Read the model definition and answer for the solid it produces. Units are mm, in the model's axes. A direction names the side the tool comes from. Give positions to 0.01 mm unless a question says otherwise; leave off trailing zeros. Order: outer loops, then holes, each group sorted by start corner. A loop starts at its lowest first (then second) coordinate and runs counter-clockwise, first axis right, second up. Notation, with made-up numbers: M 17,86 L 30,86 A20 ccw 30,109 Z; hole C -35,-11 d11. An arc over 180 degrees is marked long. Write item = value, one per line. Start each with the question number.
from build123d import *

# Parameters (mm, degrees)
SKETCH1_R           = 38.1
SKETCH1_R_2         = 34.671
BOSS_EXTRUDE1_DEPTH = 12.7
SKETCH2_W           = 12.7
SKETCH2_H           = 12.7
BOSS_EXTRUDE2_DEPTH = 12.7
SKETCH4_W           = 2.54
SKETCH4_H           = 58.988343485
CUT_EXTRUDE2_DEPTH  = 65.340360647
BOSS_EXTRUDE3_REACH = 104.44
BOSS_EXTRUDE3_START = 38.1
SKETCH5_W           = 50.267106623
SKETCH5_H           = 12.7
SKETCH6_W           = 36.83
SKETCH6_H           = 50.8
BOSS_EXTRUDE4_DEPTH = 12.7
SKETCH7_R           = 3.429
SKETCH7_W           = 10.16
SKETCH7_H           = 11.43
CUT_EXTRUDE3_DEPTH  = 109.754126547
SKETCH8_W           = 36.83
SKETCH8_H           = 12.7
CUT_EXTRUDE4_DEPTH  = 109.754126547


with BuildPart() as part:
    # Sketch1 → Boss-Extrude1 (new body)
    with BuildSketch(Plane(origin=(0, 0, 0), x_dir=(1, 0, 0), z_dir=(0, 1, 0))):
        with Locations(Location((0, 0, 0), (0, 0, 270))):
            Circle(SKETCH1_R)
        with Locations(Location((0, 0, 0), (0, 0, 270))):
            Circle(SKETCH1_R_2, mode=Mode.SUBTRACT)
    extrude(amount=BOSS_EXTRUDE1_DEPTH)

    # Sketch2 → Boss-Extrude2 (add)
    with BuildSketch(Plane(origin=(0, 0, 0), x_dir=(1, 0, 0), z_dir=(0, 1, 0))):
        with Locations((0, 43.917106623)):
            Rectangle(SKETCH2_W, SKETCH2_H)
    extrude(amount=BOSS_EXTRUDE2_DEPTH)

    # Sketch4 → Cut-Extrude2 (cut, through all)
    with BuildSketch(Plane(origin=(0, 0, 0), x_dir=(1, 0, 0), z_dir=(0, 1, 0))):
        with Locations((0, 30.925816426)):
            Rectangle(SKETCH4_W, SKETCH4_H)
    extrude(amount=CUT_EXTRUDE2_DEPTH, mode=Mode.SUBTRACT)

    # Sketch5 → Boss-Extrude3 (add, up to next)
    with BuildSketch(Plane(origin=(0, 0, 0), x_dir=(0, 0, -1), z_dir=(1, 0, 0)).offset(BOSS_EXTRUDE3_START), mode=Mode.PRIVATE) as boss_extrude3_sk1:
        with Locations((25.133553312, 6.35)):
            Rectangle(SKETCH5_W, SKETCH5_H)
    boss_extrude3_tool1 = extrude(boss_extrude3_sk1.sketch, amount=-BOSS_EXTRUDE3_REACH, mode=Mode.PRIVATE) - part.part
    add(boss_extrude3_tool1.solids().sort_by_distance((38.1, 6.35, -25.133553))[0])

    # Sketch6 → Boss-Extrude4 (add)
    with BuildSketch(Plane(origin=(0, 12.7, 0), x_dir=(1, 0, 0), z_dir=(0, 1, 0))):
        with Locations((19.685, 75.667106623)):
            Rectangle(SKETCH6_W, SKETCH6_H)
    extrude(amount=-BOSS_EXTRUDE4_DEPTH)

    # Sketch7 → Cut-Extrude3 (cut, through all)
    with BuildSketch(Plane(origin=(0, 0, 0), x_dir=(1, 0, 0), z_dir=(0, 1, 0))):
        with Locations(Location((7.62, 94.717106623, 0), (0, 0, 270))):
            Circle(SKETCH7_R)
        with Locations(Location((20.32, 94.717106623, 0), (0, 0, 270))):
            Circle(SKETCH7_R)
        with Locations(Location((20.32, 82.017106623, 0), (0, 0, 270))):
            Circle(SKETCH7_R)
        with Locations(Location((7.62, 82.017106623, 0), (0, 0, 270))):
            Circle(SKETCH7_R)
        with Locations(Location((7.62, 69.317106623, 0), (0, 0, 270))):
            Circle(SKETCH7_R)
        with Locations(Location((20.32, 69.317106623, 0), (0, 0, 270))):
            Circle(SKETCH7_R)
        with Locations(Location((7.62, 56.617106623, 0), (0, 0, 270))):
            Circle(SKETCH7_R)
        with Locations(Location((20.32, 56.617106623, 0), (0, 0, 270))):
            Circle(SKETCH7_R)
        with Locations(Location((33.02, 94.717106623, 0), (0, 0, 270))):
            Circle(SKETCH7_R)
        with Locations(Location((33.02, 82.017106623, 0), (0, 0, 270))):
            Circle(SKETCH7_R)
        with Locations(Location((33.02, 69.317106623, 0), (0, 0, 270))):
            Circle(SKETCH7_R)
        with Locations(Location((33.02, 56.617106623, 0), (0, 0, 270))):
            Circle(SKETCH7_R)
        with Locations((11.43, 43.282106623)):
            Rectangle(SKETCH7_W, SKETCH7_H)
    extrude(amount=CUT_EXTRUDE3_DEPTH, mode=Mode.SUBTRACT)

    # Sketch8 → Cut-Extrude4 (cut, through all)
    with BuildSketch(Plane(origin=(0, 12.7, 0), x_dir=(1, 0, 0), z_dir=(0, 1, 0))):
        with Locations((19.685, 94.717106623)):
            Rectangle(SKETCH8_W, SKETCH8_H)
    extrude(amount=-CUT_EXTRUDE4_DEPTH, mode=Mode.SUBTRACT)


solid = part.part
1) Find section D-D on x = 20.32. Determine the outline of the cut face in (y, z).
2) Find section A-A on y = 2. Count the separate pieces of the cut face and the enclosed holes in it, plus the area to 3 significant figures.
3) Each of these flat-tipped pins is pushed along its axis until it touches: P1, Ø5.5, axis at x = 33.02, z = -56.62, coming from the +Y side; P2, Ø11, axis at x = 33.02, z = -69.32, coming from the +Y side; P3, Ø1, axis at x = -20.5, y = 3.5, coming from the +Z side; P4, Ø3, axis at x = 11.5, y = 7.5, coming from the +Z side. Where does it stop, or does it pass through?
4) For faces 4 (the face through (11, 6, -48.997)), 5 (the face through (1.27, 6, -61)), 6 (the face through (-4, 6, -50.267)), determine the directions among +Z, -Z, +X, -X, +Y, -Y from which every point of the face is accessible in a straight line to the end or side of a thin tool.
5) Find the intervals of material crossed by probe 1 along Z at (x, y) = (4.5, 7.5); probe 2 along Z at (x, y) = (7.62, 5.5); probe 3 along X at (y, z) = (3.5, -15.5), in increasing order. Write a range as [from, to].
6) Find section C-C on x = 28. Determine the outline of the cut face in (y, z), plus the area to 3 significant figures.
7) For a pull along X with two mould halves and no side action, classify faces 1 (the face through (18.234, 6.261, -59.338)), 2 (the face through (17, 12.7, -44)), 3 (the face through (-25.51, 6.26, 28.3)) as pulls with the +X half, pulls with the -X half, needs draft (parallel to the pull), parting line crosses it, or undercut.
8) Find section B-B on z = 9. Determine the outline of the cut face in (x, y).
Numbers:
q1.outline = M 0,-88.37 L 12.7,-88.37 L 12.7,-85.45 L 0,-85.45 Z; M 0,-78.59 L 12.7,-78.59 L 12.7,-72.75 L 0,-72.75 Z; M 0,-65.89 L 12.7,-65.89 L 12.7,-60.05 L 0,-60.05 Z; M 0,-53.19 L 12.7,-53.19 L 12.7,-28.09 L 0,-28.09 Z; M 0,28.09 L 12.7,28.09 L 12.7,32.23 L 0,32.23 Z
q2.separate_pieces = 1
q2.enclosed_holes = 10
q2.area = 2,550 mm2
q3.P1 = through
q3.P2 = 12.7
q3.P3 = 32.43
q3.P4 = 36.76
q4.face_4 = +Y, -Y
q4.face_5 = -Z, +Y, -Y
q4.face_6 = -Z, -X, +Y, -Y
q5.probe_1 = [-88.37, -83.44], [-80.59, -70.74], [-67.89, -58.04], [-55.19, -34.38], [34.38, 37.83]
q5.probe_2 = [-88.37, -85.45], [-78.59, -72.75], [-65.89, -60.05], [-53.19, -49], [-37.57, -33.82], [33.82, 37.33]
q5.probe_3 = [-34.8, -31.01], [31.01, 38.1]
q6.outline = M 0,-88.37 L 12.7,-88.37 L 12.7,-20.45 L 0,-20.45 Z; M 0,20.45 L 12.7,20.45 L 12.7,25.84 L 0,25.84 Z
q6.area = 931 mm2
q7.face_1 = undercut
q7.face_2 = needs draft
q7.face_3 = parting line crosses it
q8.outline = M -37.02,0 L -33.48,0 L -33.48,12.7 L -37.02,12.7 Z; M 33.48,0 L 37.02,0 L 37.02,12.7 L 33.48,12.7 Z
